```python
from build123d import *

# Parameters (mm, degrees)
BOSS_EXTRUDE1_DEPTH   = 35
BOSS_EXTRUDE1_2_DEPTH = 35
SKETCH2_W             = 162.732130767
SKETCH2_H             = 113.961013526
BOSS_EXTRUDE2_DEPTH   = 10
SKETCH3_R             = 17.5
BOSS_EXTRUDE3_DEPTH   = 54.006142336
CUT_EXTRUDE2_REACH    = 327.764
SKETCH4_R             = 15
FILLET1_R             = 2
FILLET2_R             = 10


with BuildPart() as part:
    # Sketch1 → Boss-Extrude1 (new body)
    with BuildSketch(Plane.XY):
        Polygon((285.66695455, 30.421117945), (61.771160065, 30.421117945), (0, 84.427260281), (285.66695455, 84.427260281), align=None)
    extrude(amount=BOSS_EXTRUDE1_DEPTH)



with BuildPart() as body_2:
    # Sketch1 → Boss-Extrude1 2 (new body)
    with BuildSketch(Plane.XY):
        Polygon((28.135943206, -0.578882055), (162.732130767, -0.578882055), (162.732130767, -29.533753245), (0, -29.533753245), (0, 0), (0, 9.421117945), (28.135943206, 9.421117945), align=None)
    extrude(amount=BOSS_EXTRUDE1_2_DEPTH)


with BuildPart() as part_1:
    add(part.part)

    add(body_2.part)  # Boss-Extrude2 merges body 2
    # Sketch2 → Boss-Extrude2 (add)
    with BuildSketch(Plane(origin=(0, 0, 0), x_dir=(-1, 0, 0), z_dir=(0, 0, -1))):
        with Locations((-81.366065384, 27.446753518)):
            Rectangle(SKETCH2_W, SKETCH2_H)
    extrude(amount=BOSS_EXTRUDE2_DEPTH)

    # Sketch3 → Boss-Extrude3 (add)
    with BuildSketch(Plane(origin=(0, 84.427260281, 0), x_dir=(1, 0, 0), z_dir=(0, 1, 0))):
        with Locations((285.66695455, -17.5)):
            Circle(SKETCH3_R)
    extrude(amount=-BOSS_EXTRUDE3_DEPTH)

    # Sketch4 → Cut-Extrude2 (cut, up to next)
    with BuildSketch(Plane(origin=(0, 84.427260281, 0), x_dir=(1, 0, 0), z_dir=(0, 1, 0)), mode=Mode.PRIVATE) as cut_extrude2_sk1:
        with Locations(Location((285.66695455, -17.5, 0), (0, 0, 270))):
            Circle(SKETCH4_R)
    cut_extrude2_tool1 = extrude(cut_extrude2_sk1.sketch, amount=-CUT_EXTRUDE2_REACH, mode=Mode.PRIVATE) & part_1.part
    add(cut_extrude2_tool1.solids().sort_by_distance((285.666955, 84.42726, 17.5))[0], mode=Mode.SUBTRACT)

    # Fillet1
    fillet1_edges = [part_1.edges().sort_by_distance(p)[0] for p in [
        (0, 9.421117945, 17.5),
        (28.135943206, 9.421117945, 17.5),
        (28.135943206, -0.578882055, 17.5),
    ]]
    fillet(fillet1_edges, radius=FILLET1_R)

    # Fillet2
    fillet2_edges = [part_1.edges().sort_by_distance(p)[0] for p in [
        (162.732130767, -0.578882055, 17.5),
        (61.771160065, 30.421117945, 17.5),
    ]]
    fillet(fillet2_edges, radius=FILLET2_R)


solid = part_1.part
```
The listing builds one solid part. Answer for the finished solid, in the listing's coordinates (mm). A direction names the side the tool comes from. Coordinates: 2 decimals unless noted, no trailing zeros. Write each loop counter-clockwise with the first axis right and the second up, starting at its lowest first coordinate (ties: lowest second). Pieces come first, ordered by that corner, then holes. Notation, with made-up numbers: M 69.25,13 L 117.25,13 A25 ccw 117.25,38 Z; hole C 37.25,4.5 d1. An arc over 180 degrees is marked long. Use a Markdown table: item, result. Add a question column.
1. Which of the six approach directions +Z, -Z, +X, -X, +Y, -Y give full straight-line access (tool end or side, diameter ignored) to faces 5 (the flat face through (162.732, 1, -2)), 6 (the flat face through (183, 30.421, 17)), 7 (the cylindrical face through (62.06, 31.04, 17.74))?
2. Straight lines are drawn through the part: line 1 along Y through (x, z) = (108.5, 17); line 2 along Z through (x, y) = (162.5, -4); line 3 along X through (y, z) = (61, 18). For each, find the intervals that lie inside material, in ascending order. Write a range as [from, to].
3. Section D-D (z = 5.5) is taken. Give the vertices of the cut face in (x, y).
4. Section B-B (x = 98.5) is taken. Give the vertices of the cut face in (y, z).
5. Section A-A (z = 17.5) is taken. Give the vertices of the cut face in (x, y), plus the area to 3 significant figures.
6. Given P1, Ø3, axis at x = 245, z = 25.5, coming from the -Y side; P2, Ø1, axis at y = 40.5, z = 21, coming from the +X side; P3, Ø1.8, axis at y = 3.5, z = 26, coming from the +X side, each flat-ended and moving along its own axis, determine where each tip first touches the part or whether it passes through.
7. For a pull along X with two mould halves and no side action, classify faces 1 (the flat face through (0, 1, 8)), 2 (the cylindrical face through (271.024, 57.802, 14.248)), 3 (the cylindrical face through (159.725, -3.43, 17.745)), 4 (the flat face through (225, 58, 0)) as +X half, -X half, draft (parallel to the pull), parting line (faces both ways), or undercut.
8. Section C-C (y = 57.5) is taken. Give the vertices of the cut face in (x, z).
Data:
| question | item | result |
|---|---|---|
| 1 | face 5 | -Z, +X, -Y |
| 1 | face 6 | +Z, +X, -X |
| 1 | face 7 | +Z, -X |
| 2 | line 1 | y = [-29.53, -0.58], [30.42, 84.43] |
| 2 | line 2 | z = [-10, 0] |
| 2 | line 3 | x = [26.8, 270.68], [300.66, 303.16] |
| 3 | outline | M 0,-29.53 L 162.73,-29.53 L 162.73,-10.58 A10 ccw 152.73,-0.58 L 30.14,-0.58 A2 cw 28.14,1.42 L 28.14,7.42 A2 ccw 26.14,9.42 L 2,9.42 A2 ccw 0,7.42 Z; M 0,84.43 L 58.94,32.89 A10 ccw 65.53,30.42 L 276.67,30.42 L 276.67,84.43 Z; M 294.67,30.42 L 298.4,30.42 L 298.4,84.43 L 294.67,84.43 Z |
| 4 | outline | M -29.53,-10 L 84.43,-10 L 84.43,35 L 30.42,35 L 30.42,0 L -0.58,0 L -0.58,35 L -29.53,35 Z |
| 5 | outline | M 0,-29.53 L 162.73,-29.53 L 162.73,-10.58 A10 ccw 152.73,-0.58 L 30.14,-0.58 A2 cw 28.14,1.42 L 28.14,7.42 A2 ccw 26.14,9.42 L 2,9.42 A2 ccw 0,7.42 Z; M 0,84.43 L 58.94,32.89 A10 ccw 65.53,30.42 L 270.67,30.42 L 270.67,84.43 Z; M 300.67,30.42 L 303.17,30.42 L 303.17,84.43 L 300.67,84.43 Z |
| 5 | area | 18,100 mm2 |
| 6 | P1 | stops at y = 30.42 |
| 6 | P2 | stops at x = 302.91 |
| 6 | P3 | stops at x = 28.14 |
| 7 | face 1 | -X half |
| 7 | face 2 | undercut |
| 7 | face 3 | +X half |
| 7 | face 4 | draft |
| 8 | outline | M 0,-10 L 162.73,-10 L 162.73,0 L 285.67,0 A17.5 ccw 285.67,35 L 30.8,35 L 30.8,0 L 0,0 Z; hole C 285.67,17.5 d30 |
